```python
from build123d import *

# Parameters (mm, degrees)
F1_DEPTH = 12.5
F2_R     = 10


with BuildPart() as f1:
    # F0 (on Front) → F1 (new body, symmetric)
    with BuildSketch(Plane.XZ):
        with BuildLine():
            Line((350, 230), (40.9729498071, 230))
            add(Edge.make_bspline(
                [(40.9729498071, 230), (23.1266754436, 217.7466324391), (9.1600259417, 205)],
                knots=[5.8517425134, 5.8517425134, 5.8517425134, 5.949769397, 5.949769397, 5.949769397], degree=2, weights=[1, 0.9987990817, 1]))
            Line((9.1600259417, 205), (350, 205))
            Line((350, 205), (350, 230))
        make_face()
        with BuildLine():
            add(Edge.make_bspline(
                [(-68.7509398502, 115), (-68.7509398502, 55.2165740433), (0, 0)],
                knots=[0, 0, 0, 0.393402632, 0.393402632, 0.393402632], degree=2, weights=[1, 0.9807165918, 1]))
            Line((0, 0), (28.125, 0))
            Line((28.125, 0), (40.9729498071, 0))
            add(Edge.make_bspline(
                [(9.1600259417, 25), (23.1266754436, 12.2533675609), (40.9729498071, 0)],
                knots=[0.3334159102, 0.3334159102, 0.3334159102, 0.4314427937, 0.4314427937, 0.4314427937], degree=2, weights=[1, 0.9987990817, 1]))
            add(Edge.make_bspline(
                [(-38.7509398502, 115), (-38.7509398502, 68.7258392336), (9.1600259417, 25)],
                knots=[0, 0, 0, 0.3334159102, 0.3334159102, 0.3334159102], degree=2, weights=[1, 0.9861363811, 1]))
            add(Edge.make_bspline(
                [(9.1600259417, 205), (-38.7509398502, 161.2741607664), (-38.7509398502, 115)],
                knots=[5.949769397, 5.949769397, 5.949769397, 6.2831853072, 6.2831853072, 6.2831853072], degree=2, weights=[1, 0.9861363811, 1]))
            add(Edge.make_bspline(
                [(40.9729498071, 230), (23.1266754436, 217.7466324391), (9.1600259417, 205)],
                knots=[5.8517425134, 5.8517425134, 5.8517425134, 5.949769397, 5.949769397, 5.949769397], degree=2, weights=[1, 0.9987990817, 1]))
            Line((40.9729498071, 230), (0, 230))
            add(Edge.make_bspline(
                [(0, 230), (-68.7509398502, 174.7834259567), (-68.7509398502, 115)],
                knots=[5.8897826752, 5.8897826752, 5.8897826752, 6.2831853072, 6.2831853072, 6.2831853072], degree=2, weights=[1, 0.9807165918, 1]))
        make_face()
        with BuildLine():
            add(Edge.make_bspline(
                [(9.1600259417, 25), (23.1266754436, 12.2533675609), (40.9729498071, 0)],
                knots=[0.3334159102, 0.3334159102, 0.3334159102, 0.4314427937, 0.4314427937, 0.4314427937], degree=2, weights=[1, 0.9987990817, 1]))
            Line((40.9729498071, 0), (59.1832854123, 0))
            Line((59.1832854123, 0), (620, 0))
            Line((620, 0), (620, 25))
            Line((620, 25), (9.1600259417, 25))
        make_face()
        with BuildLine():
            Line((40.9729498071, 0), (28.125, 0))
            Line((28.125, 0), (23.4899694027, -17.2981696839))
            add(Edge.make_bspline(
                [(23.4899694027, -17.2981696839), (35.9947939251, -25.7814361907), (50.0769032841, -33.9854807757)],
                knots=[0.4567057683, 0.4567057683, 0.4567057683, 0.5196982713, 0.5196982713, 0.5196982713], degree=2, weights=[1, 0.9995040341, 1]))
            Line((50.0769032841, -33.9854807757), (56.4775823084, -10.0978214541))
            add(Edge.make_bspline(
                [(40.9729498071, 0), (48.3992260092, -5.0989293373), (56.4775823084, -10.0978214541)],
                knots=[0.4314427937, 0.4314427937, 0.4314427937, 0.4722612324, 0.4722612324, 0.4722612324], degree=2, weights=[1, 0.9997917391, 1]))
        make_face()
        with BuildLine():
            add(Edge.make_bspline(
                [(23.4899694027, -17.2981696839), (35.9947939251, -25.7814361907), (50.0769032841, -33.9854807757)],
                knots=[0.4567057683, 0.4567057683, 0.4567057683, 0.5196982713, 0.5196982713, 0.5196982713], degree=2, weights=[1, 0.9995040341, 1]))
            Line((23.4899694027, -17.2981696839), (-54.9392496536, -310))
            Line((-54.9392496536, -310), (-23.8809642413, -310))
            Line((-23.8809642413, -310), (50.0769032841, -33.9854807757))
        make_face()
        with BuildLine():
            Line((59.1832854123, 0), (40.9729498071, 0))
            add(Edge.make_bspline(
                [(40.9729498071, 0), (48.3992260092, -5.0989293373), (56.4775823084, -10.0978214541)],
                knots=[0.4314427937, 0.4314427937, 0.4314427937, 0.4722612324, 0.4722612324, 0.4722612324], degree=2, weights=[1, 0.9997917391, 1]))
            Line((56.4775823084, -10.0978214541), (59.1832854123, 0))
        make_face()
    extrude(amount=F1_DEPTH, both=True)

    # F2
    f2_edges = [f1.edges().sort_by_distance(p)[0] for p in [
        (9.160026, 6.25, 25),
        (9.160026, -6.25, 25),
        (9.160026, 6.25, 205),
        (9.160026, -6.25, 205),
        (59.183285, 0, 0),
        (28.125, 0, 0),
    ]]
    fillet(f2_edges, radius=F2_R)


solid = f1.part
```
For this review, take the finished solid that the model builds, in its own axes (mm). A direction names the side the tool comes from. Round coordinates to 2 decimals unless told otherwise and drop trailing zeros. Write each loop counter-clockwise with the first axis right and the second up, starting at its lowest first coordinate (ties: lowest second). Pieces come first, ordered by that corner, then holes. Notation, with made-up numbers: (-14, 10.5) -> (5, 10.5) arc R12 ccw to (5, 27.5) -> close; hole circle Ø5 at (28.5, 64). An arc over 180 degrees is marked (long way). Use one line per item in the form item = value.
Q1. To check wall thickness, follow probe 1 along Z at (x, y) = (73.5, 9.75); probe 2 along Z at (x, y) = (559.5, 8.75); probe 3 along X at (y, z) = (-5, 97). State the ranges of each line that lie inside material, in increasing order. Write a range as from..to.
Resolved:
probe_1 = 0..25, 205..230
probe_2 = 0..25
probe_3 = -67.13..-36.89
Q2. Consider section A-A (x = 193.5). State the section outline as (y, z) points, then the cut area to 3 significant figures.
Resolved:
outline = (-12.5, 0) -> (12.5, 0) -> (12.5, 25) -> (-12.5, 25) -> close; (-12.5, 205) -> (12.5, 205) -> (12.5, 230) -> (-12.5, 230) -> close
area = 1,250 mm²
Q3. Clearance check with flat-ended pins moving along their axes: pin 1 Ø5 at (y, z) = (-9, -171) entering from +X; pin 2 Ø12.5 at (x, y) = (345.5, 3) entering from -Z; pin 3 Ø12 at (y, z) = (-1, 60) entering from +X. State where each tip first meets the part, or that it passes through.
Resolved:
pin_1 = 14.03
pin_2 = 0
pin_3 = -17.08
Q4. The part is to be moulded in two halves that separate along Z. For faces 6 (the flat face through (321, 0, 25)), 7 (the flat face through (177, 0, 230)), 8 (the flat face through (340, 0, 0)), 9 (the flat face through (172, 12.5, 21)), say which applies: released by +Z, released by -Z, zero draft, split by the parting line, or undercut.
Resolved:
face_6 = undercut
face_7 = released by +Z
face_8 = released by -Z
face_9 = zero draft
Q5. Consider section C-C (x = 424.5). State the section outline as (y, z) points, then the cut area to 3 significant figures.
Resolved:
outline = (-12.5, 0) -> (12.5, 0) -> (12.5, 25) -> (-12.5, 25) -> close
area = 625 mm²
Q6. Consider section B-B (z = -251). State the section outline as (x, y) points, then the cut area to 3 significant figures.
Resolved:
outline = (-39.13, -12.5) -> (-8.07, -12.5) -> (-8.07, 12.5) -> (-39.13, 12.5) -> close
area = 776 mm²
Q7. Machinability: for faces 1 (the flat face through (-40, 0, -310)), 2 (the flat face through (7, 0, 0)), 3 (the flat face through (350, 0, 217)), 4 (the flat face through (179, 0, 205)), 5 (the flat face through (620, 0, 12)), which of the approach directions +Z, -Z, +X, -X, +Y, -Y give a long, thin tool a straight path to every point of the face, cutting with its end or side? Answer none if there is none.
Resolved:
face_1 = -Z, +X, -X, +Y, -Y
face_2 = -X, +Y, -Y
face_3 = +Z, +X, +Y, -Y
face_4 = +X, +Y, -Y
face_5 = +Z, -Z, +X, +Y, -Y
